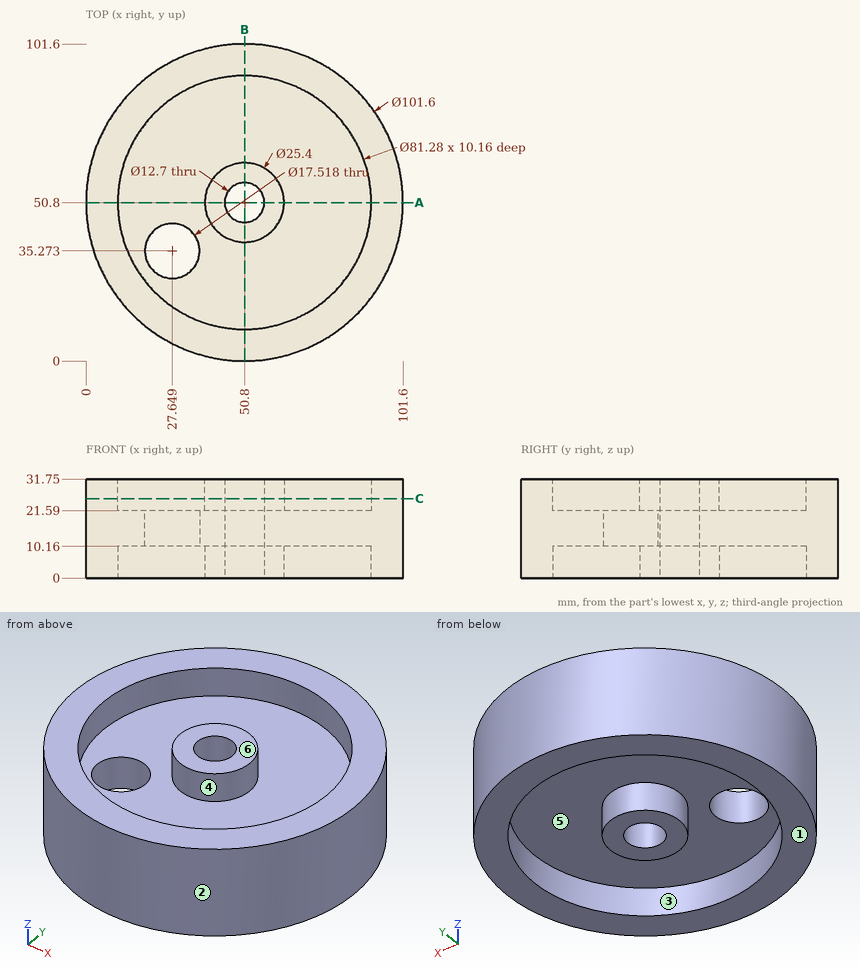
Study the drawing (mm; zero at the part's minimum x, y, z) and answer. A direction names the side the tool comes from. Give positions to 0.01 mm unless a question says otherwise; leave off trailing zeros. Order: outer loops, then holes, each group sorted by start corner. A loop starts at its lowest first (then second) coordinate and runs counter-clockwise, first axis right, second up. Notation, with made-up numbers: (27.5, -20.75) - (39.5, -20.75) arc R26 ccw to (39.5, 15.25) - close; hole circle Ø7 at (37, -23). An arc over 180 degrees is marked (long way). Use one line per item in the form item = value. Start each with the question number.
(1) Flat-ended cylindrical pins translate along their axes: pin 1 Ø7.5 at (x, y) = (50.8, 50.8) entering from -Z; pin 2 Ø10 at (y, z) = (63, 17.5) entering from +X; pin 3 Ø12 at (y, z) = (10.5, 4.5) entering from -X; pin 4 Ø10 at (x, z) = (82.5, 14.5) entering from +Y. Find the tip coordinate at first contact, or state that the pin passes through.
(2) The mould has two halves that part along Y. Classify the marked faces 1, 2 and 3: released by +Y, released by -Y, zero draft, split by the parting line, or undercut.
(3) A cutting plane is placed at A-A, the plane y = 50.8. Write down the section's boundary in (x, z).
(4) A cutting plane is placed at C-C, the plane z = 25.5. Write down the section's boundary in (x, y), then the cut area to 3 significant figures.
(5) For the marked faces 4, 5 and 6, determine the directions among +Z, -Z, +X, -X, +Y, -Y from which every point of the face is accessible in a straight line to the end or side of a thin tool.
(6) Consider line 1 (Y direction, x = 50.8, z = 23.5); line 2 (Y direction, x = 46.5, z = 24.5); line 3 (Y direction, x = 57.5, z = 30) (1 decimal). Determine where each line is inside the solid, lowest interval first. Write a range as from..to.
Ans:
q1.pin_1 = through
q1.pin_2 = 101.09
q1.pin_3 = 13.33
q1.pin_4 = 94.02
q2.face_1 = zero draft
q2.face_2 = split by the parting line
q2.face_3 = undercut
q3.outline = (0, 0) - (10.16, 0) - (10.16, 10.16) - (38.1, 10.16) - (38.1, 0) - (44.45, 0) - (44.45, 31.75) - (38.1, 31.75) - (38.1, 21.59) - (10.16, 21.59) - (10.16, 31.75) - (0, 31.75) - close; (57.15, 0) - (63.5, 0) - (63.5, 10.16) - (91.44, 10.16) - (91.44, 0) - (101.6, 0) - (101.6, 31.75) - (91.44, 31.75) - (91.44, 21.59) - (63.5, 21.59) - (63.5, 31.75) - (57.15, 31.75) - close
q4.outline = circle Ø101.6 at (50.8, 50.8); circle Ø25.4 at (50.8, 50.8); hole circle Ø81.28 at (50.8, 50.8); hole circle Ø12.7 at (50.8, 50.8)
q4.area = 3,300 mm^2
q5.face_4 = +Z
q5.face_5 = -Z
q5.face_6 = +Z, +X, -X, +Y, -Y
q6.line_1 = 0..10.16, 38.1..44.45, 57.15..63.5, 91.44..101.6
q6.line_2 = 0.18..10.39, 38.85..46.13, 55.47..62.75, 91.21..101.42
q6.line_3 = 0.4..10.7, 40..61.6, 90.9..101.2
